Could you check a few things on this model? Use its own coordinates, in mm. A direction names the side the tool comes from. Round coordinates to 2 decimals unless told otherwise and drop trailing zeros. Loops run counter-clockwise (first coordinate to the right, second up) from the corner with the lowest first, then second, coordinate; pieces in that order, holes last. Notation, with made-up numbers: (58, 54.25) - (93, 54.25) arc R23 ccw to (93, 87.25) - close; hole circle Ø11 at (17.25, 50.5). An arc over 180 degrees is marked (long way). Use one line per item in the form item = value.
```python
from build123d import *

# Parameters (mm, degrees)
BOSS_EXTRUDE1_DEPTH = 0.7
BOSS_EXTRUDE2_DEPTH = 5
FILLET1_R           = 5
FILLET2_R           = 2


with BuildPart() as part:
    # Sketch1 → Boss-Extrude1 (new body)
    with BuildSketch(Plane.XY):
        Polygon((0, 71), (0, 0), (34.4076055, 0), (34.4076055, 16), (55.4076055, 16), (55.4076055, 23.5), (77.4076055, 23.5), (77.4076055, 16), (130.4076055, 16), (130.4076055, 0), (164.815211, 0), (164.815211, 71), align=None)
        Polygon((47.233378, 65), (54.483378, 47.6), (54.483378, 36.6), (47.233378, 54), align=None, mode=Mode.SUBTRACT)
        Polygon((67.233378, 65), (67.233378, 54), (59.983378, 36.6), (59.983378, 47.6), align=None, mode=Mode.SUBTRACT)
        Polygon((71.472387, 65), (78.722387, 47.6), (78.722387, 36.6), (71.472387, 54), align=None, mode=Mode.SUBTRACT)
        Polygon((57.233378, 53), (52.233378, 65), (62.233378, 65), align=None, mode=Mode.SUBTRACT)
        Polygon((81.472387, 53), (76.472387, 65), (86.472387, 65), align=None, mode=Mode.SUBTRACT)
        Polygon((91.472387, 65), (91.472387, 54), (84.222387, 36.6), (84.222387, 47.6), align=None, mode=Mode.SUBTRACT)
        Polygon((95.711396, 65), (102.961396, 47.6), (102.961396, 36.6), (95.711396, 54), align=None, mode=Mode.SUBTRACT)
        Polygon((115.711396, 65), (115.711396, 54), (108.461396, 36.6), (108.461396, 47.6), align=None, mode=Mode.SUBTRACT)
        Polygon((105.711396, 53), (100.711396, 65), (110.711396, 65), align=None, mode=Mode.SUBTRACT)
    extrude(amount=BOSS_EXTRUDE1_DEPTH)

    # Sketch1_4 → Boss-Extrude2 (add)
    with BuildSketch(Plane.XY):
        Polygon((153.923863, 64.75), (149.298863, 53.65), (144.673863, 64.75), align=None)
        Polygon((146.298863, 47.55), (146.298863, 37.85), (139.548863, 54.05), (139.548863, 63.75), align=None)
        Polygon((152.298863, 47.55), (159.048863, 63.75), (159.048863, 54.05), (152.298863, 37.85), align=None)
        Polygon((20.141348, 64.75), (15.516348, 53.65), (10.891348, 64.75), align=None)
        Polygon((12.516348, 37.85), (5.766348, 54.05), (5.766348, 63.75), (12.516348, 47.55), align=None)
        Polygon((18.516348, 37.85), (18.516348, 47.55), (25.266348, 63.75), (25.266348, 54.05), align=None)
    extrude(amount=-BOSS_EXTRUDE2_DEPTH)

    # Fillet1
    fillet1_edges = [part.edges().sort_by_distance(p)[0] for p in [
        (34.4076055, 16, 0.35),
        (34.4076055, 0, 0.35),
        (130.4076055, 0, 0.35),
        (130.4076055, 16, 0.35),
    ]]
    fillet(fillet1_edges, radius=FILLET1_R)

    # Fillet2
    fillet2_edges = [part.edges().sort_by_distance(p)[0] for p in [
        (77.4076055, 23.5, 0.35),
        (55.4076055, 23.5, 0.35),
        (55.4076055, 16, 0.35),
        (77.4076055, 16, 0.35),
    ]]
    fillet(fillet2_edges, radius=FILLET2_R)


solid = part.part
```
1. If we section it at C-C, the plane y = 25: Write out the boundary of the cut face in (x, z), plus the area to 3 significant figures.
Solution:
outline = (0, 0) - (164.82, 0) - (164.82, 0.7) - (0, 0.7) - close
area = 115 mm^2
2. If we section it at A-A, the plane z = -1.4: Write out the boundary of the cut face in (x, y).
Solution:
outline = (5.77, 54.05) - (12.52, 37.85) - (12.52, 47.55) - (5.77, 63.75) - close; (10.89, 64.75) - (15.52, 53.65) - (20.14, 64.75) - close; (18.52, 37.85) - (25.27, 54.05) - (25.27, 63.75) - (18.52, 47.55) - close; (139.55, 54.05) - (146.3, 37.85) - (146.3, 47.55) - (139.55, 63.75) - close; (144.67, 64.75) - (149.3, 53.65) - (153.92, 64.75) - close; (152.3, 37.85) - (159.05, 54.05) - (159.05, 63.75) - (152.3, 47.55) - close
3. If we section it at D-D, the plane y = 51: Count the separate pieces of the cut face and the enclosed holes in it, plus the area to 3 significant figures.
Solution:
separate_pieces = 7
enclosed_holes = 0
area = 177 mm^2
4. For P1, Ø2.5, axis at y = 41.5, z = -1.5, coming from the +X side; P2, Ø0.6, axis at x = 97, z = 0.5, coming from the -Y side; P3, Ø2, axis at x = 69.5, y = 60.5, coming from the -Z side, each with a flat end and sliding along its axis, tell me the tip position at first contact or that it passes through.
Solution:
P1 = 154.34
P2 = 16
P3 = 0
5. We'd pull the mould along X, two halves only. Please class faces 1 (the face through (159.049, 59, -2)), 2 (the face through (143, 51, -5)), 3 (the face through (50.9, 45.2, 0.3)): +X half, -X half, draft (parallel to the pull), parting line (faces both ways), or undercut.
Solution:
face_1 = +X half
face_2 = draft
face_3 = undercut
6. If we section it at B-B, the plane y = 13: Write out the boundary of the cut face in (x, z), plus the area to 3 significant figures.
Solution:
outline = (0, 0) - (34.83, 0) - (34.83, 0.7) - (0, 0.7) - close; (129.99, 0) - (164.82, 0) - (164.82, 0.7) - (129.99, 0.7) - close
area = 48.8 mm^2
7. On a 3-axis mill with a long thin cutter (end or side, diameter ignored), from which of +Z, -Z, +X, -X, +Y, -Y can I reach the whole of each face in a straight line? I mean faces 4 (the face through (149, 64.75, -2)), 5 (the face through (155.63, 55.54, -2.46)), 6 (the face through (59.768, 59.084, 0.345)), 7 (the face through (131.911, 1.426, 0.355)). Say none if no direction works.
Solution:
face_4 = -Z, +X, -X, +Y
face_5 = -Z
face_6 = +Z, -Z
face_7 = +Z, -Z, -Y
8. Please list where these lines run through material, in increasing order: line 1 along X through (y, z) = (57, -2.7); line 2 along X through (y, z) = (56.5, -3.25); line 3 along Z through (x, y) = (68, 54.5).
Solution:
line_1 = 5.77 to 8.58, 14.12 to 16.91, 22.45 to 25.27, 139.55 to 142.36, 147.9 to 150.69, 156.24 to 159.05
line_2 = 5.77 to 8.79, 14.33 to 16.7, 22.25 to 25.27, 139.55 to 142.57, 148.11 to 150.49, 156.03 to 159.05
line_3 = 0 to 0.7
